Autodesk Inventor part; units mm, degrees
ref_plane "YZ Plane" through (0, 0, 0) normal (1, 0, 0) x (0, 1, 0)
ref_plane "XZ Plane" through (0, 0, 0) normal (0, 1, 0) x (-1, 0, 0)
ref_plane "XY Plane" through (0, 0, 0) normal (0, 0, 1) x (1, 0, 0)
sketch "Sketch1" plane through (0, 0, 0) normal (0, 0, 1) x (1, 0, 0)
  line L0 (-10, -10) -> (10, -10)
  line L1 (10, -10) -> (10, 10)
  line L2 (10, 10) -> (-10, 10)
  line L3 (-10, 10) -> (-10, -10)
  line L4 (-10, -10) -> (10, 10) construction
  line L5 (10, -10) -> (-10, 10) construction
  line L6 (-7.25, -7.25) -> (7.25, -7.25)
  line L7 (7.25, -7.25) -> (7.25, 7.25)
  line L8 (7.25, 7.25) -> (-7.25, 7.25)
  line L9 (-7.25, 7.25) -> (-7.25, -7.25)
  line L10 (-7.25, -7.25) -> (7.25, 7.25) construction
  line L11 (7.25, -7.25) -> (-7.25, 7.25) construction
  point P0 (0, 0)
  dimension "d0" = 20
  dimension "d1" = 20
  dimension "d2" = 14.5
  dimension "d3" = 14.5
extrude "Extrusion1" add sketch "Sketch1" along normal blind 1000
equation "\"d3\" = d2"
properties part number "aluprofile_1m" material "Aluminum 6061"
Read the model definition and answer for the solid it produces. Units are mm, in the model's axes. Give positions to 0.01 mm unless a question says otherwise; leave off trailing zeros. Write each loop counter-clockwise with the first axis right and the second up, starting at its lowest first coordinate (ties: lowest second). Pieces come first, ordered by that corner, then holes. Notation, with made-up numbers: (37, 29) -> (59, 29) arc R24 ccw to (59, 56) -> close; hole circle Ø10 at (5.25, 49.5). An arc over 180 degrees is marked (long way). Answer in a Markdown table with one row per item.
1) Section C-C on z = 857 is taken. Give the vertices of the cut face in (x, y), plus the area to 3 significant figures.
Results list:
| item | result |
|---|---|
| outline | (-10, -10) -> (10, -10) -> (10, 10) -> (-10, 10) -> close; hole (-7.25, -7.25) -> (7.25, -7.25) -> (7.25, 7.25) -> (-7.25, 7.25) -> close |
| area | 190 mm^2 |
2) A straight line is drawn through the part: line 1 (X direction, y = 5, z = 883). Find the intervals that lie inside material, in ascending order. Write a range as [from, to].
Results list:
| item | result |
|---|---|
| line 1 | [-10, -7.25], [7.25, 10] |
3) Section A-A on x = 1.5 is taken. Give the vertices of the cut face in (y, z), plus the area to 3 significant figures.
Results list:
| item | result |
|---|---|
| outline | (-10, 0) -> (-7.25, 0) -> (-7.25, 1000) -> (-10, 1000) -> close; (7.25, 0) -> (10, 0) -> (10, 1000) -> (7.25, 1000) -> close |
| area | 5,500 mm^2 |
